Could you check a few things on this drawing? It's one solid part, dimensions in mm from its lowest x, y, z. Give positions to 0.01 mm unless a question says otherwise; leave off trailing zeros. Order: outer loops, then holes, each group sorted by start corner. A loop starts at its lowest first (then second) coordinate and runs counter-clockwise, first axis right, second up. Notation, with made-up numbers: M 79,51.5 L 108,51.5 A17 cw 108,81.5 Z; hole C 84,34.25 d2. An arc over 180 degrees is marked long. One line per item, written item: value. Start each with the question number.
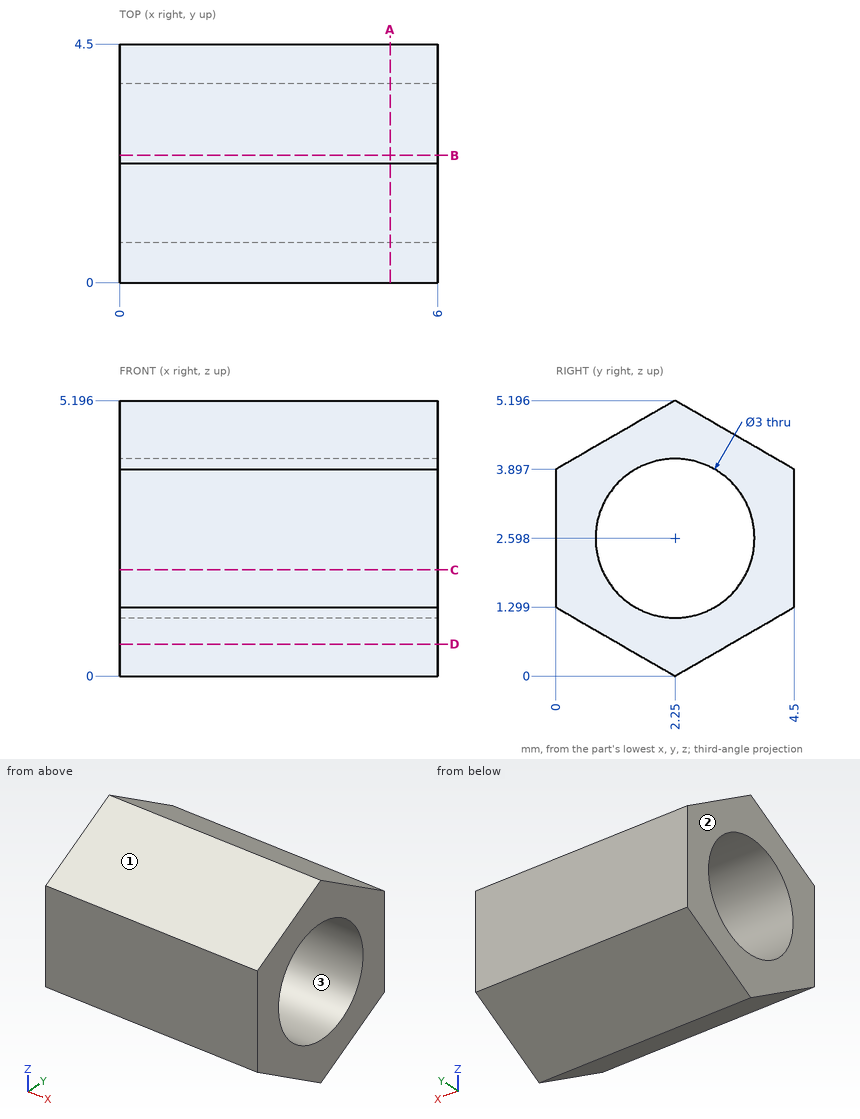
Item 1: I want a section at A-A on x = 5.1. Write out the boundary of the cut face in (y, z).
Item 2: I want a section at B-B on y = 2.4. Write out the boundary of the cut face in (x, z), plus the area to 3 significant figures.
Item 3: I want a section at C-C on z = 2. Write out the boundary of the cut face in (x, y).
Item 4: We'd pull the mould along Y, two halves only. Please class the marked faces 1, 2 and 3: +Y half, -Y half, draft (parallel to the pull), parting line (faces both ways), or undercut.
Item 5: I want a section at D-D on z = 0.6. Write out the boundary of the cut face in (x, y), plus the area to 3 significant figures.
Item 6: Will these pins go through, and if not, where does the flat tip stop? P1, Ø2.5, axis at y = 2.25, z = 2.6, coming from the +X side; P2, Ø1.5, axis at x = 2, y = 4, coming from the +Z side; P3, Ø1, axis at x = 3.5, y = 0.5, coming from the -Z side.
Item 7: Please list where these lines run through material, in increasing order: probe 1 along Y at (x, z) = (4.55, 2.65); probe 2 along Z at (x, y) = (0.95, 2.95) (1 decimal); probe 3 along Z at (x, y) = (2.25, 1.75). Write a range as [from, to].
Answer below:
1. outline: M 0,1.3 L 2.25,0 L 4.5,1.3 L 4.5,3.9 L 2.25,5.2 L 0,3.9 Z; hole C 2.25,2.6 d3
2. outline: M 0,0.09 L 6,0.09 L 6,1.11 L 0,1.11 Z; M 0,4.09 L 6,4.09 L 6,5.11 L 0,5.11 Z
2. area: 12.2 mm²
3. outline: M 0,0 L 6,0 L 6,0.87 L 0,0.87 Z; M 0,3.63 L 6,3.63 L 6,4.5 L 0,4.5 Z
4. face 1: -Y half
4. face 2: draft
4. face 3: undercut
5. outline: M 0,1.21 L 6,1.21 L 6,3.29 L 0,3.29 Z
5. area: 12.5 mm²
6. P1: passes through
6. P2: stops at z = 4.62
6. P3: stops at z = 0.72
7. probe 1: y = [0, 0.75], [3.75, 4.5]
7. probe 2: z = [0.4, 1.3], [3.9, 4.8]
7. probe 3: z = [0.29, 1.18], [4.01, 4.91]
